The drawing under review shows one solid part. Ordinate dimensions are in mm from its lowest x, y, z. Coordinates: 2 decimals unless noted, no trailing zeros. Loops run counter-clockwise (first coordinate to the right, second up) from the corner with the lowest first, then second, coordinate; pieces in that order, holes last. Notation, with made-up numbers: M -27,28.25 L -20,28.25 A32 ccw -20,55.25 Z; hole C 34,35 d4. An arc over 180 degrees is marked long. Return JSON: item names as keys, results as strings.
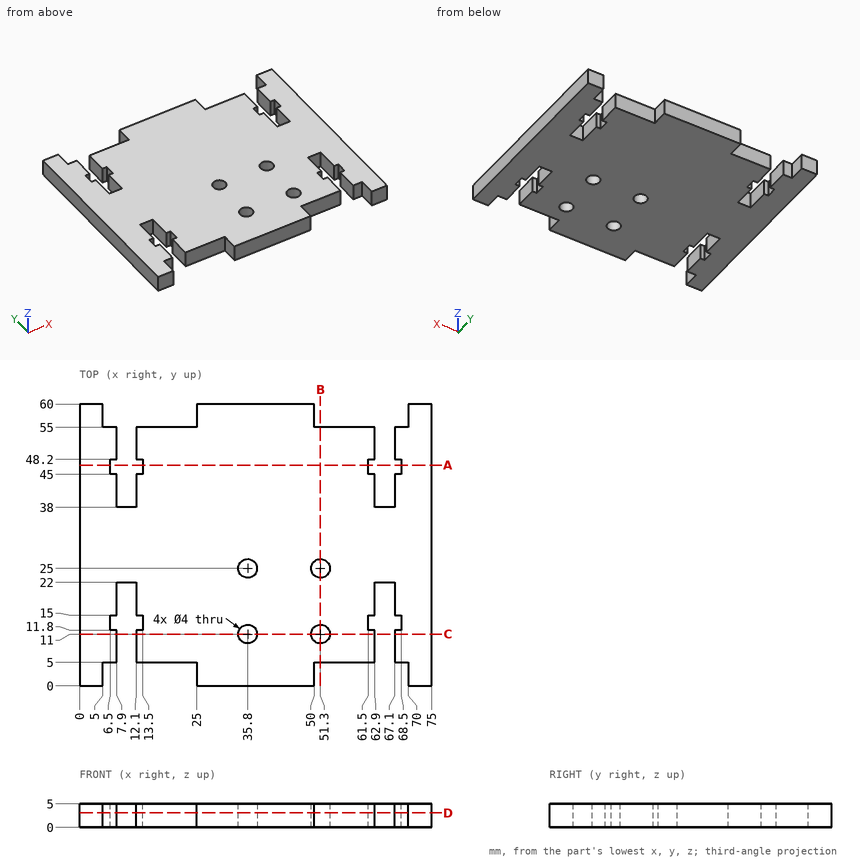
1. Add section A-A on y = 47. Give the boundary of the cut face in (x, z), plus the area to 3 significant figures.
Check values:
{"outline": "M 0,0 L 6.5,0 L 6.5,5 L 0,5 Z; M 13.5,0 L 61.5,0 L 61.5,5 L 13.5,5 Z; M 68.5,0 L 75,0 L 75,5 L 68.5,5 Z", "area": "305 mm²"}
2. Add section B-B on x = 51.3. Give the boundary of the cut face in (y, z), plus the area to 3 significant figures.
Check values:
{"outline": "M 5,0 L 9,0 L 9,5 L 5,5 Z; M 13,0 L 23,0 L 23,5 L 13,5 Z; M 27,0 L 55,0 L 55,5 L 27,5 Z", "area": "210 mm²"}
3. Add section C-C on y = 11. Give the boundary of the cut face in (x, z).
Check values:
{"outline": "M 0,0 L 7.9,0 L 7.9,5 L 0,5 Z; M 12.1,0 L 33.8,0 L 33.8,5 L 12.1,5 Z; M 37.8,0 L 49.3,0 L 49.3,5 L 37.8,5 Z; M 53.3,0 L 62.9,0 L 62.9,5 L 53.3,5 Z; M 67.1,0 L 75,0 L 75,5 L 67.1,5 Z"}
4. To check wall thickness, follow line 1 (X direction, y = 48, z = 4.25); line 2 (Y direction, x = 35.8, z = 1.85); line 3 (X direction, y = 39.5, z = 0.85). State the ranges of each line that lie inside material, in increasing order.
Check values:
{"line 1": "0 to 6.5, 13.5 to 61.5, 68.5 to 75", "line 2": "0 to 9, 13 to 23, 27 to 60", "line 3": "0 to 7.9, 12.1 to 62.9, 67.1 to 75"}
5. Add section D-D on z = 3.05. State how many separate pieces and enclosed holes the cut face has, plus the area to 3 significant figures.
Check values:
{"separate pieces": "1", "enclosed holes": "4", "area": "3,730 mm²"}
6. Insertion check: pin 1 Ø1.5 at (x, z) = (13, 2) entering from -Y; pin 2 Ø2 at (x, z) = (64, 2.5) entering from -Y; pin 3 Ø1.5 at (x, z) = (7, 3) entering from +Y. Each pin has a flat end and moves straight along its axis. Give the tip position at first contact, or say it passes through.
Check values:
{"pin 1": "y = 5", "pin 2": "y = 22", "pin 3": "y = 55"}
